```python
from build123d import *

# Parameters (mm, degrees)
SKETCH1_W           = 250
SKETCH1_H           = 150
BOSS_EXTRUDE1_DEPTH = 6.35
SKETCH2_R           = 2.5
SKETCH2_W           = 30
SKETCH2_H           = 95
CUT_EXTRUDE1_DEPTH  = 146.912036858
FILLET1_R           = 10
SKETCH3_R           = 2
CUT_EXTRUDE2_DEPTH  = 146.912036858


with BuildPart() as part:
    # Sketch1 → Boss-Extrude1 (new body)
    with BuildSketch(Plane(origin=(0, 0, 0), x_dir=(1, 0, 0), z_dir=(0, 1, 0))):
        Rectangle(SKETCH1_W, SKETCH1_H)
    extrude(amount=BOSS_EXTRUDE1_DEPTH)

    # Sketch2 → Cut-Extrude1 (cut, through all)
    with BuildSketch(Plane(origin=(0, 6.35, 0), x_dir=(1, 0, 0), z_dir=(0, 1, 0))):
        with Locations(Location((-115, 65, 0), (0, 0, 270))):
            Circle(SKETCH2_R)
        with Locations(Location((115, 65, 0), (0, 0, 270))):
            Circle(SKETCH2_R)
        with Locations(Location((115, -65, 0), (0, 0, 270))):
            Circle(SKETCH2_R)
        with Locations(Location((-115, -65, 0), (0, 0, 270))):
            Circle(SKETCH2_R)
        Rectangle(SKETCH2_W, SKETCH2_H)
    extrude(amount=-CUT_EXTRUDE1_DEPTH, mode=Mode.SUBTRACT)

    # Fillet1
    fillet1_edges = [part.edges().sort_by_distance(p)[0] for p in [
        (-15, 3.175, 47.5),
        (-15, 3.175, -47.5),
        (15, 3.175, -47.5),
        (15, 3.175, 47.5),
        (-125, 3.175, -75),
        (125, 3.175, -75),
        (125, 3.175, 75),
        (-125, 3.175, 75),
    ]]
    fillet(fillet1_edges, radius=FILLET1_R)

    # Sketch3 → Cut-Extrude2 (cut, through all)
    with BuildSketch(Plane(origin=(0, 6.35, 0), x_dir=(1, 0, 0), z_dir=(0, 1, 0))):
        with Locations(Location((-60.62, 35, 0), (0, 0, 270))):
            Circle(SKETCH3_R)
        with Locations(Location((-60.62, -10, 0), (0, 0, 270))):
            Circle(SKETCH3_R)
        with Locations(Location((-60.62, -55, 0), (0, 0, 270))):
            Circle(SKETCH3_R)
        with Locations(Location((60.62, 35, 0), (0, 0, 270))):
            Circle(SKETCH3_R)
        with Locations(Location((60.62, -10, 0), (0, 0, 270))):
            Circle(SKETCH3_R)
        with Locations(Location((60.62, -55, 0), (0, 0, 270))):
            Circle(SKETCH3_R)
        with Locations(Location((-26.5, 27.5, 0), (0, 0, 270))):
            Circle(SKETCH3_R)
        with Locations(Location((-26.5, -27.5, 0), (0, 0, 270))):
            Circle(SKETCH3_R)
        with Locations(Location((26.5, -27.5, 0), (0, 0, 270))):
            Circle(SKETCH3_R)
        with Locations(Location((26.5, 27.5, 0), (0, 0, 270))):
            Circle(SKETCH3_R)
        with Locations(Location((-26.5, 0, 0), (0, 0, 270))):
            Circle(SKETCH3_R)
        with Locations(Location((26.5, 0, 0), (0, 0, 270))):
            Circle(SKETCH3_R)
    extrude(amount=-CUT_EXTRUDE2_DEPTH, mode=Mode.SUBTRACT)


solid = part.part
```
Read the model definition and answer for the solid it produces. Units are mm, in the model's axes. A direction names the side the tool comes from. Round coordinates to 2 decimals unless told otherwise and drop trailing zeros. Write each loop counter-clockwise with the first axis right and the second up, starting at its lowest first coordinate (ties: lowest second). Pieces come first, ordered by that corner, then holes. Notation, with made-up numbers: M 22.5,6 L 57.5,6 A17 cw 57.5,33 Z; hole C 38.5,42 d7. An arc over 180 degrees is marked long. One line per item, written item: value.
Q1. Find section B-B on z = -15. Write down the section's boundary in (x, y).
Data:
outline: M -125,0 L -15,0 L -15,6.35 L -125,6.35 Z; M 15,0 L 125,0 L 125,6.35 L 15,6.35 Z
Q2. For a pull along Z with two mould halves and no side action, classify faces 3 (the cylindrical face through (117.48, 3.22, 64.67)), 4 (the cylindrical face through (-122.15, 3.22, 71.99)), 5 (the flat face through (-30, 6.35, -1)), 6 (the cylindrical face through (-122.15, 3.22, -71.99)) as +Z half, -Z half, draft (parallel to the pull), parting line (faces both ways), or undercut.
Data:
face 3: undercut
face 4: +Z half
face 5: draft
face 6: -Z half
Q3. Find section A-A on y = 2.75. Count the separate pieces of the cut face and the enclosed holes in it, plus the area to 3 significant figures.
Data:
separate pieces: 1
enclosed holes: 17
area: 34,400 mm2
Q4. Straight lines are drawn through the part: line 1 (X direction, y = 3.5, z = 10); line 2 (X direction, y = 2.75, z = 55); line 3 (X direction, y = 1.5, z = 27.5). For each, find the intervals that lie inside material, in ascending order. Write a range as [from, to].
Data:
line 1: [-125, -62.62], [-58.62, -15], [15, 58.62], [62.62, 125]
line 2: [-125, -62.62], [-58.62, 58.62], [62.62, 125]
line 3: [-125, -28.5], [-24.5, -15], [15, 24.5], [28.5, 125]
Q5. Flat-ended cylindrical pins translate along their axes: pin 1 Ø6.5 at (x, z) = (26.5, 0) entering from -Y; pin 2 Ø4.5 at (x, z) = (-115, 65) entering from -Y. Find the tip coordinate at first contact, or state that the pin passes through.
Data:
pin 1: y = 0
pin 2: through
Q6. Which of the six approach directions +Z, -Z, +X, -X, +Y, -Y give full straight-line access (tool end or side, diameter ignored) to faces 1 (the flat face through (-2, 3, -75)), 2 (the cylindrical face through (11.99, 3.13, 44.65))?
Data:
face 1: -Z, +X, -X, +Y, -Y
face 2: +Y, -Y
